from build123d import *

# Parameters (mm, degrees)
LOFT1_START        = -0.9525
LOFT1_DEPTH        = 1.905
CUT_EXTRUDE2_DEPTH = 110.33494104
SKETCH5_R          = 7.3025
CUT_EXTRUDE3_DEPTH = 108.939694094


with BuildPart() as part:
    # Loft1: read off the stored shape, not the designer's step
    # Loft1 outline → Loft1 (new body)
    with BuildSketch(Plane(origin=(0, 0, 0), x_dir=(1, 0, 0), z_dir=(0, 1, 0)).offset(LOFT1_START)):
        with BuildLine():
            add(Edge.make_bspline(
                [(0, -15.875), (21.314656151, -21.106845313), (57.417925413, -25.838728987), (92.603989484, -17.720178647), (106.934, -10.795)],
                knots=[0, 0, 0, 0, 0.588632913, 1, 1, 1, 1], degree=3))
            Line((106.934, -10.795), (106.934, 10.795))
            add(Edge.make_bspline(
                [(0, 15.875), (21.314656151, 21.106845313), (57.417925413, 25.838728987), (92.603989484, 17.720178647), (106.934, 10.795)],
                knots=[0, 0, 0, 0, 0.588632913, 1, 1, 1, 1], degree=3))
            Line((0, 15.875), (0, -15.875))
        make_face()
    extrude(amount=LOFT1_DEPTH)

    # Sketch4 → Cut-Extrude2 (cut, through all)
    with BuildSketch(Plane(origin=(0, 0.9525, 0), x_dir=(1, 0, 0), z_dir=(0, 1, 0))):
        with BuildLine():
            Line((0, 15.875), (0, 3e-09))
            ThreePointArc((0, 3e-09), (2.975795104, 7.184204898), (10.16, 10.16))
            Line((10.16, 10.16), (21.188013281, 10.16))
            ThreePointArc((21.188013281, 10.16), (22.845695922, 10.268650261), (24.475015153, 10.592742006))
            Line((24.475015153, 10.592742006), (37.72679711, 14.14354628))
            ThreePointArc((37.72679711, 14.14354628), (40.05104351, 14.539743655), (42.408472673, 14.499476682))
            Line((42.408472673, 14.499476682), (99.60820705, 8.179760764))
            ThreePointArc((99.60820705, 8.179760764), (104.834824793, 5.490348999), (106.934, 0))
            Line((106.934, 0), (106.934, 10.795))
            add(Edge.make_bspline(
                [(0, 15.875), (21.314656151, 21.106845313), (57.417925413, 25.838728987), (92.603989484, 17.720178647), (106.934, 10.795)],
                knots=[0, 0, 0, 0, 0.588632913, 1, 1, 1, 1], degree=3))
        make_face()
        with BuildLine():
            Line((21.188013281, -10.16), (10.16, -10.16))
            ThreePointArc((10.16, -10.16), (2.975795102, -7.184204896), (0, 3e-09))
            Line((0, 3e-09), (0, -15.875))
            add(Edge.make_bspline(
                [(0, -15.875), (21.314656151, -21.106845313), (57.417925413, -25.838728987), (92.603989484, -17.720178647), (106.934, -10.795)],
                knots=[0, 0, 0, 0, 0.588632913, 1, 1, 1, 1], degree=3))
            Line((106.934, -10.795), (106.934, 0))
            ThreePointArc((106.934, 0), (104.834824793, -5.490348999), (99.60820705, -8.179760764))
            Line((99.60820705, -8.179760764), (42.408472673, -14.499476682))
            ThreePointArc((42.408472673, -14.499476682), (40.05104351, -14.539743655), (37.72679711, -14.14354628))
            Line((37.72679711, -14.14354628), (24.475015153, -10.592742006))
            ThreePointArc((24.475015153, -10.592742006), (22.845695922, -10.268650261), (21.188013281, -10.16))
        make_face()
    extrude(amount=-CUT_EXTRUDE2_DEPTH, mode=Mode.SUBTRACT)

    # Sketch5 → Cut-Extrude3 (cut, through all)
    with BuildSketch(Plane(origin=(0, 0.9525, 0), x_dir=(1, 0, 0), z_dir=(0, 1, 0))):
        with Locations(Location((10.16, 0, 0), (0, 0, 270))):
            Circle(SKETCH5_R)
    extrude(amount=-CUT_EXTRUDE3_DEPTH, mode=Mode.SUBTRACT)

    # Mirror1: part across plane


with BuildPart() as part_1:
    add(part.part)
    add(part.part.mirror(Plane(origin=(10.16, 0, 0), x_dir=(0, 0, 1), z_dir=(1, 0, 0))))


solid = part_1.part
The listing builds one solid part. Answer for the finished solid, in the listing's coordinates (mm). A direction names the side the tool comes from. Give positions to 0.01 mm unless a question says otherwise; leave off trailing zeros. Loops run counter-clockwise (first coordinate to the right, second up) from the corner with the lowest first, then second, coordinate; pieces in that order, holes last. Notation, with made-up numbers: (23, -7.5) - (27, -7.5) arc R27 cw to (27, 13.5) - close; hole circle Ø2 at (-26.5, 41). An arc over 180 degrees is marked (long way). Answer as a JSON object with one key per item and string values.
1. A cutting plane is placed at D-D (x = 71). Write down the section's boundary in (y, z).
Determined:
{"outline": "(-0.95, -11.34) - (0.95, -11.34) - (0.95, 11.34) - (-0.95, 11.34) - close"}
2. A cutting plane is placed at A-A (y = 0.1). Write down the section's boundary in (x, z) (1 decimal).
Determined:
{"outline": "(-79.3, -8.2) - (-22.1, -14.5) arc R12.7 ccw to (-17.4, -14.1) - (-4.2, -10.6) arc R12.7 cw to (-0.9, -10.2) - (21.2, -10.2) arc R12.7 cw to (24.5, -10.6) - (37.7, -14.1) arc R12.7 ccw to (42.4, -14.5) - (99.6, -8.2) arc R8.2 ccw to (99.6, 8.2) - (42.4, 14.5) arc R12.7 ccw to (37.7, 14.1) - (24.5, 10.6) arc R12.7 cw to (21.2, 10.2) - (-0.9, 10.2) arc R12.7 cw to (-4.2, 10.6) - (-17.4, 14.1) arc R12.7 ccw to (-22.1, 14.5) - (-79.3, 8.2) arc R8.2 ccw to start; hole circle Ø14.6 at (10.2, 0)"}
3. A cutting plane is placed at B-B (x = 10.16). Write down the section's boundary in (y, z), then the cut area to 3 significant figures.
Determined:
{"outline": "(-0.95, -10.16) - (0.95, -10.16) - (0.95, -7.3) - (-0.95, -7.3) - close; (-0.95, 7.3) - (0.95, 7.3) - (0.95, 10.16) - (-0.95, 10.16) - close", "area": "10.9 mm²"}
4. For a pull along Z with two mould halves and no side action, classify faces 4 (the flat face through (-51.089, 0.013, 11.295)), 5 (the flat face through (70.608, 0.013, -11.384)), 6 (the cylindrical face through (3.03, 0.01, -1.58)) as pulls with the +Z half, pulls with the -Z half, needs draft (parallel to the pull), parting line crosses it, or undercut.
Determined:
{"face 4": "pulls with the +Z half", "face 5": "pulls with the -Z half", "face 6": "undercut"}
5. Find the intervals of material crossed by L1, parallel to X at y = 0.3, z = 4.5; L2, parallel to Z at x = 4, y = -0.45; L3, parallel to X at y = 0.65, z = 3.25, in increasing order. Write a range as [from, to].
Determined:
{"L1": "[-85.27, 4.41], [15.91, 105.59]", "L2": "[-10.16, -3.92], [3.92, 10.16]", "L3": "[-85.95, 3.62], [16.7, 106.27]"}
6. Flat-ended cylindrical pins translate along their axes: pin 1 Ø4 at (x, z) = (7, 2.5) entering from -Y; pin 2 Ø0.6 at (x, y) = (7.5, 0) entering from -Z. Find the tip coordinate at first contact, or state that the pin passes through.
Determined:
{"pin 1": "through", "pin 2": "z = -10.16"}
7. For faces 1 (the flat face through (31.19, 0.01, 12.39)), 2 (the flat face through (9, -0.952, 10)), 3 (the flat face through (31.008, 0.013, -12.343)), determine the directions among +Z, -Z, +X, -X, +Y, -Y from which every point of the face is accessible in a straight line to the end or side of a thin tool.
Determined:
{"face 1": "+Z, +Y, -Y", "face 2": "+Z, -Z, +X, -X, -Y", "face 3": "-Z, +Y, -Y"}
8. A cutting plane is placed at C-C (z = -3). Write down the section's boundary in (x, y).
Determined:
{"outline": "(-86.05, -0.95) - (3.5, -0.95) - (3.5, 0.95) - (-86.05, 0.95) - close; (16.82, -0.95) - (106.37, -0.95) - (106.37, 0.95) - (16.82, 0.95) - close"}
